Could you check a few things on this drawing? It's one solid part, dimensions in mm from its lowest x, y, z. Coordinates: 2 decimals unless noted, no trailing zeros. Loops run counter-clockwise (first coordinate to the right, second up) from the corner with the lowest first, then second, coordinate; pieces in that order, holes last.
1) If I drill on line 1 along X through (y, z) = (30, 0.65); line 2 along Y through (x, z) = (65, 0.3); line 3 along X through (y, z) = (66.44, 1.05), over which ranges is the centre line in solid material (lowest first)?
2) Will these pins go through, and if not, where does the flat tip stop? P1, Ø2.5, axis at x = 75, y = 66.44, coming from the +Z side; P2, Ø0.8, axis at x = 99.5, z = 0.5, coming from the +Y side.
3) Imagine slicing it at A-A on z = 0.9. Please give me the cut outline in (x, y).
4) Imagine slicing it at C-C on y = 37.5. Please give me the cut outline in (x, z).
5) Imagine slicing it at B-B on x = 94. Please give me the cut outline in (y, z), plus the area to 3 significant figures.
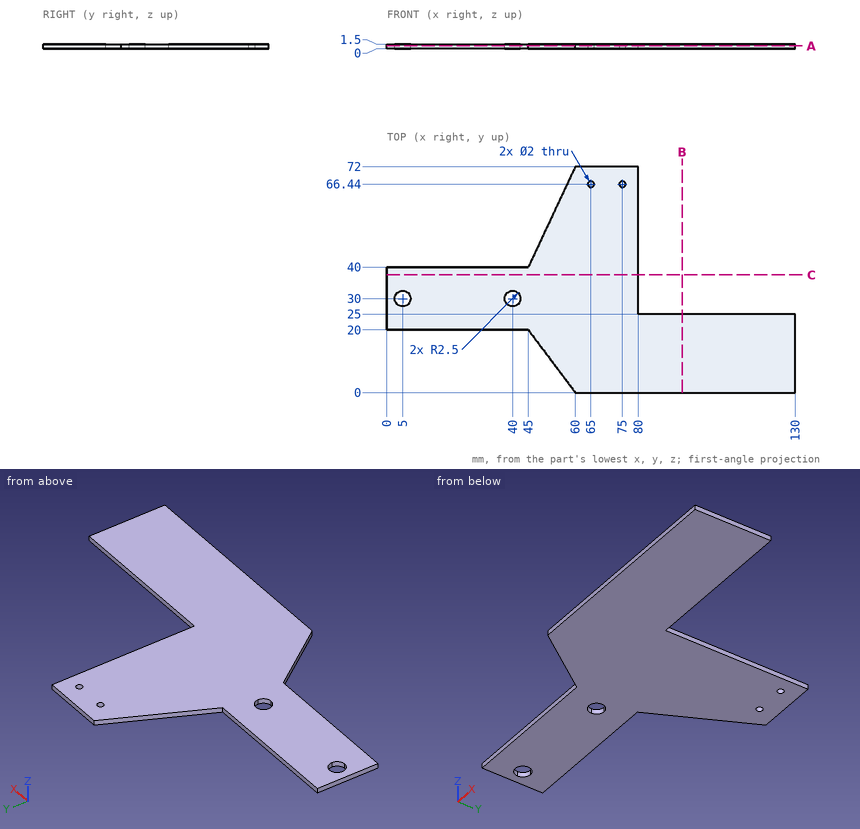
Filled in:
1. line 1: x = 0 to 2.5, 7.5 to 37.5, 42.5 to 80
1. line 2: y = 0 to 65.44, 67.44 to 72
1. line 3: x = 57.39 to 64, 66 to 74, 76 to 80
2. P1: stops at z = 1.5
2. P2: stops at y = 25
3. outline: (0, 20) - (45, 20) - (60, 0) - (130, 0) - (130, 25) - (80, 25) - (80, 72) - (60, 72) - (45, 40) - (0, 40) - close; hole circle Ø5 at (5, 30); hole circle Ø5 at (40, 30); hole circle Ø2 at (65, 66.44); hole circle Ø2 at (75, 66.44)
4. outline: (0, 0) - (80, 0) - (80, 1.5) - (0, 1.5) - close
5. outline: (0, 0) - (25, 0) - (25, 1.5) - (0, 1.5) - close
5. area: 37.5 mm2
